Geometry: final body of the model. Coordinates: model frame, mm. A direction names the side the tool comes from. Coordinates: 2 decimals unless noted, no trailing zeros. Loops run counter-clockwise (first coordinate to the right, second up) from the corner with the lowest first, then second, coordinate; pieces in that order, holes last. Notation, with made-up numbers: (79, 87.25) - (130, 87.25) arc R20 cw to (130, 125.25) - close; hole circle Ø7 at (-20, 42.25). An arc over 180 degrees is marked (long way). Return JSON: item names as keys, results as strings.
Autodesk Inventor part; units mm, degrees
ref_plane "YZ Plane" through (0, 0, 0) normal (1, 0, 0) x (0, 1, 0)
ref_plane "XZ Plane" through (0, 0, 0) normal (0, 1, 0) x (-1, 0, 0)
ref_plane "XY Plane" through (0, 0, 0) normal (0, 0, 1) x (1, 0, 0)
sketch "Sketch1" plane through (0, 0, 0) normal (0, 0, 1) x (1, 0, 0)
  line L0 (-56, 0) -> (-28, 48.4974)
  line L1 (-28, 48.4974) -> (28, 48.4974)
  line L2 (28, 48.4974) -> (56, 0)
  line L3 (56, 0) -> (28, -48.4974)
  line L4 (28, -48.4974) -> (-28, -48.4974)
  line L5 (-28, -48.4974) -> (-56, 0)
  circle A0 centre (0, 30) radius 2.5
  circle A1 centre (-25.9808, 15) radius 2.5
  circle A2 centre (-25.9808, -15) radius 2.5
  circle A3 centre (0, -30) radius 2.5
  circle A4 centre (25.9808, -15) radius 2.5
  circle A5 centre (25.9808, 15) radius 2.5
  point P0 (0, 0)
  point P1 (0, 0)
  dimension "d0" = 112
  dimension "d1" = 5
  dimension "d2" = 30
  dimension "d5" = 360
extrude "Extrusion1" add sketch "Sketch1" along normal blind 5
sketch "Sketch2" plane through (0, 0, 5) normal (0, 0, 1) x (1, 0, 0)
  line L0 (28, 48.4974) -> (-28, 48.4974)
  line L1 (28, 48.4974) -> (128, 48.4974)
  line L2 (128, 48.4974) -> (128, -48.4974)
  line L3 (128, -48.4974) -> (28, -48.4974)
  circle A0 centre (25.9808, 15) radius 2.5
  circle A1 centre (25.9808, -15) radius 2.5
  line L4 (56, 0) -> (28, 48.4974)
  line L5 (28, -48.4974) -> (56, 0)
  line L6 (-28, -48.4974) -> (28, -48.4974)
  line L7 (28, -48.4974) -> (56, 0)
  line L8 (28, 48.4974) -> (56, 0)
  line L9 (28, -48.4974) -> (128, -48.4974)
  line L10 (28, 48.4974) -> (128, 48.4974)
  point P0 (0, 0)
  dimension "d10" = 100
extrude "Extrusion2" add sketch "Sketch2" against normal blind 5 contours L1 L2 L3 L5 L4
sketch "Sketch3" plane through (128, -48.4974, 5) normal (1, 0, 0) x (0, 0, -1)
  line L0 (0, 0) -> (0, 96.9948)
  line L1 (-58, 96.9948) -> (-30, 48.4974)
  line L2 (-30, 48.4974) -> (-58, 0)
  line L3 (-58, 0) -> (-114, 0)
  line L4 (-114, 0) -> (-142, 48.4974)
  line L5 (-142, 48.4974) -> (-114, 96.9948)
  line L6 (-114, 96.9948) -> (-58, 96.9948)
  line L7 (0, 0) -> (-58, 0)
  line L8 (-58, 0) -> (-58, 96.9948) construction
  line L9 (-58, 96.9948) -> (0, 96.9948)
  line L10 (0, 96.9948) -> (0, 0)
  circle A0 centre (-86, 78.4974) radius 2.5
  circle A1 centre (-111.9808, 63.4974) radius 2.5
  circle A2 centre (-111.9808, 33.4974) radius 2.5
  circle A3 centre (-86, 18.4974) radius 2.5
  circle A4 centre (-60.0192, 33.4974) radius 2.5
  circle A5 centre (-60.0192, 63.4974) radius 2.5
  line L11 (-58, 0) -> (-30, 48.4974)
  line L12 (-30, 48.4974) -> (-58, 96.9948)
  line L13 (-58, 96.9948) -> (0, 96.9948)
  line L14 (0, 48.4974) -> (0, 0)
  line L15 (-58, 0) -> (0, 0)
  circle A6 centre (-86, 48.4974) radius 22.5
  point P0 (5, 48.4974)
  dimension "d17" = 112
  dimension "d18" = 30
  dimension "d19" = 5
  dimension "d20" = 30
  dimension "d23" = 360
  dimension "d27" = 45
extrude "Extrusion3" add sketch "Sketch3" against normal blind 5
sketch "Sketch4" plane through (0, 0, 5) normal (0, 0, 1) x (1, 0, 0)
  circle A0 centre (0, 0) radius 22.5
  dimension "d28" = 45
extrude "Extrusion4" cut sketch "Sketch4" against normal through all
sketch "Sketch5" plane through (0, 0, 5) normal (0, 0, 1) x (1, 0, 0)
  circle A0 centre (0, 0) radius 22.5
  line L0 (123, -48.4974) -> (123, 48.4974) construction
  line L1 (123, 48.4974) -> (-28, 48.4974)
  line L2 (-28, 48.4974) -> (-56, 0)
  line L3 (-56, 0) -> (-28, -48.4974)
  line L4 (-28, -48.4974) -> (123, -48.4974)
  circle A1 centre (25.9808, 15) radius 2.5
  circle A2 centre (25.9808, -15) radius 2.5
  circle A3 centre (0, -30) radius 2.5
  circle A4 centre (-25.9808, -15) radius 2.5
  circle A5 centre (-25.9808, 15) radius 2.5
  circle A6 centre (0, 30) radius 2.5
  line L5 (-22.2265, 38.4974) -> (113, 38.4974)
  line L6 (113, 38.4974) -> (113, -38.4974) construction
  line L7 (113, -38.4974) -> (-22.2265, -38.4974)
  line L8 (-22.2265, -38.4974) -> (-44.453, 0)
  line L9 (-44.453, 0) -> (-22.2265, 38.4974)
  line L10 (113, 38.4974) -> (123, 38.4974)
  line L11 (123, -48.4974) -> (123, 48.4974)
  line L12 (123, 48.4974) -> (123, 38.4974)
  line L13 (113, -38.4974) -> (123, -38.4974)
  line L14 (123, -38.4974) -> (123, -48.4974)
  dimension "d31" = 10
extrude "Extrusion5" add sketch "Sketch5" along normal blind 15 contours L11 L10 L5 L9 L8 L7 L13 L4 L3 L2 L1
sketch "Sketch7" plane through (123, -48.4974, 5) normal (-1, 0, 0) x (0, 0, 1)
  circle A0 centre (86, 78.4974) radius 2.5
  circle A1 centre (111.9808, 63.4974) radius 2.5
  circle A2 centre (111.9808, 33.4974) radius 2.5
  circle A3 centre (86, 18.4974) radius 2.5
  circle A4 centre (60.0192, 33.4974) radius 2.5
  circle A5 centre (60.0192, 63.4974) radius 2.5
  circle A6 centre (86, 48.4974) radius 22.5
  line L0 (15, 96.9948) -> (15, 86.9948)
  line L1 (15, 86.9948) -> (0, 86.9948)
  line L2 (0, 10) -> (0, 86.9948)
  line L3 (0, 10) -> (15, 10)
  line L4 (15, 10) -> (15, 0)
  line L5 (15, 0) -> (114, 0)
  line L6 (114, 0) -> (142, 48.4974)
  line L7 (142, 48.4974) -> (114, 96.9948)
  line L8 (114, 96.9948) -> (15, 96.9948)
  line L9 (0, 55.9974) -> (15, 55.9974)
  line L10 (15, 55.9974) -> (15, 40.9974)
  line L11 (15, 40.9974) -> (0, 40.9974)
  line L12 (0, 40.9974) -> (0, 55.9974)
  point P0 (-5, 48.4974)
  point P1 (0, 48.4974)
  dimension "d34" = 15
extrude "Extrusion6" cut sketch "Sketch7" against normal through all contours L9 L10 L11 L2
sketch "Sketch8" plane through (128, -48.4974, 0) normal (1, 0, 0) x (0, 0, -1)
  line L0 (-5, 40.9974) -> (-20, 40.9974)
  line L1 (-20, 40.9974) -> (-20, 55.9974)
  line L2 (-20, 55.9974) -> (-5, 55.9974)
  line L3 (-5, 55.9974) -> (-5, 40.9974)
  circle A0 centre (-91, 78.4974) radius 2.5
  circle A1 centre (-116.9808, 63.4974) radius 2.5
  circle A2 centre (-116.9808, 33.4974) radius 2.5
  circle A3 centre (-91, 18.4974) radius 2.5
  circle A4 centre (-65.0192, 33.4974) radius 2.5
  circle A5 centre (-65.0192, 63.4974) radius 2.5
  circle A6 centre (-91, 48.4974) radius 22.5
  line L4 (-119, 0) -> (0, 0)
  line L5 (0, 96.9948) -> (0, 0)
  line L6 (0, 96.9948) -> (-119, 96.9948)
  line L7 (-119, 96.9948) -> (-147, 48.4974)
  line L8 (-147, 48.4974) -> (-119, 0)
  line L9 (-113.2265, 86.9948) -> (-10, 86.9948)
  line L10 (-10, 86.9948) -> (-10, 10) construction
  line L11 (-10, 10) -> (-113.2265, 10)
  line L12 (-113.2265, 10) -> (-135.453, 48.4974)
  line L13 (-135.453, 48.4974) -> (-113.2265, 86.9948)
  line L14 (-10, 86.9948) -> (0, 86.9948)
  line L15 (-10, 10) -> (0, 10)
  line L16 (0, 96.9948) -> (0, 0)
  point P0 (0, 48.4974)
  dimension "d37" = 10
extrude "Extrusion7" add sketch "Sketch8" along normal blind 15 contours L8 L7 L6 L5 L14 L9 L13 L12 L11 L15 L4
sketch "Sketch9" plane through (128, -38.4974, 0) normal (1, 0, 0) x (0, 0, -1)
  line L0 (0, 76.9948) -> (0, 86.9948)
  line L1 (0, 76.9948) -> (-5, 76.9948)
  line L2 (-5, 76.9948) -> (-5, -0.838)
  line L3 (-5, -0.838) -> (0, -0.838)
  line L4 (0, -0.838) -> (0, 76.9948)
  line L5 (-5, 45.9974) -> (-5, 30.9974)
  point P0 (0, 38.4974)
extrude "Extrusion8" add sketch "Sketch9" along normal blind 15
sketch "Sketch10" plane through (128, -7.5, 20) normal (1, 0, 0) x (0, 0, -1)
  circle A0 centre (7.5, 35) radius 2.5
  circle A1 centre (7.5, -20) radius 2.5
  line L0 (0, 15) -> (15, 15) construction
  line L1 (7.5, -20) -> (7.5, 35) construction
  line L2 (0, 0) -> (0, 15) construction
  point P0 (20, 7.5)
  point P1 (7.5, 15)
  point P2 (7.5, 7.5)
  point P3 (0, 7.5)
  dimension "d42" = 5
  dimension "d43" = 5
  dimension "d44" = 55
extrude "Extrusion9" cut sketch "Sketch10" against normal blind 20
sketch "Sketch12" plane through (-28, 48.4974, 20) normal (0, 1, 0) x (1, 0, 0)
  line L0 (151, 0) -> (151, -99) construction
  line L1 (151, -60) -> (91, 0)
  line L2 (151, 0) -> (5.7735, 0) construction
  line L3 (151, 15) -> (151, 0)
  line L4 (91, 0) -> (151, 0)
  line L5 (151, 0) -> (151, -60)
  point P0 (28, 20)
  dimension "d47" = 60
  dimension "d48" = 60
extrude "Extrusion10" add sketch "Sketch12" against normal blind 10
sketch "Sketch13" plane through (-28, -48.4974, 20) normal (0, -1, 0) x (1, 0, 0)
  line L0 (151, 60) -> (91, 0)
  line L1 (0, 0) -> (151, 0)
  line L2 (151, 0) -> (151, 99)
  line L3 (91, 0) -> (151, 0)
  line L4 (151, 60) -> (151, -15)
  line L5 (151, 60) -> (151, 0)
  point P0 (28, -20)
extrude "Extrusion11" add sketch "Sketch13" against normal blind 10
sketch "Sketch14" plane through (123, -48.4974, 5) normal (-1, 0, 0) x (0, 0, 1)
  circle A0 centre (86, 48.4974) radius 22.5
  line L0 (114, 96.9948) -> (142, 48.4974)
  line L1 (142, 48.4974) -> (114, 0)
  line L2 (114, 0) -> (58, 0)
  line L3 (58, 0) -> (30, 48.4974)
  line L4 (30, 48.4974) -> (58, 96.9948)
  line L5 (58, 96.9948) -> (114, 96.9948)
  line L6 (114, 96.9948) -> (142, 48.4974)
  point P0 (-5, 48.4974)
extrude "Extrusion12" cut sketch "Sketch14" along normal through all
sketch "Sketch16" plane through (143, -48.4974, 0) normal (1, 0, 0) x (0, 0, -1)
  circle A0 centre (-91, 48.4974) radius 22.5 construction
  circle A1 centre (-142, 48.4974) radius 2.5
  circle A2 centre (-116.5, 4.3301) radius 2.5
  circle A3 centre (-65.5, 4.3301) radius 2.5
  circle A4 centre (-40, 48.4974) radius 2.5
  circle A5 centre (-65.5, 92.6647) radius 2.5
  circle A6 centre (-116.5, 92.6647) radius 2.5
  point P0 (0, 48.4974)
  point P1 (-147, 48.4974)
  dimension "d55" = 5
  dimension "d56" = 5
  dimension "d59" = 360
extrude "Extrusion13" cut sketch "Sketch16" against normal through all
sketch "Sketch17" plane through (143, -48.4974, 0) normal (1, 0, 0) x (0, 0, -1)
  circle A0 centre (-142, 48.4974) radius 2.5
  circle A1 centre (-91, 48.4974) radius 22.5 construction
  circle A2 centre (-142, 48.4974) radius 6.5
  circle A3 centre (-116.5, 4.3301) radius 6.5
  circle A4 centre (-65.5, 4.3301) radius 6.5
  circle A5 centre (-40, 48.4974) radius 6.5
  circle A6 centre (-65.5, 92.6647) radius 6.5
  circle A7 centre (-116.5, 92.6647) radius 6.5
  point P0 (0, 48.4974)
  dimension "d63" = 13
  dimension "d66" = 360
extrude "Extrusion14" cut sketch "Sketch17" against normal blind 5 contours A0 | A2 | A3 | A4 | A5 | A6 | A7
sketch "Sketch18" plane through (0, 0, 20) normal (0, 0, 1) x (1, 0, 0)
  circle A0 centre (-51, 0) radius 2.5
  circle A1 centre (-25.5, -44.1673) radius 2.5
  circle A2 centre (25.5, -44.1673) radius 2.5
  circle A3 centre (51, 0) radius 2.5
  circle A4 centre (25.5, 44.1673) radius 2.5
  circle A5 centre (-25.5, 44.1673) radius 2.5
  point P0 (0, 0)
  point P1 (-56, 0)
  dimension "d70" = 5
  dimension "d71" = 5
  dimension "d74" = 360
extrude "Extrusion15" cut sketch "Sketch18" against normal through all
sketch "Sketch19" plane through (0, 0, 20) normal (0, 0, 1) x (1, 0, 0)
  circle A0 centre (-51, 0) radius 2.5
  circle A1 centre (-51, 0) radius 6.5
  circle A2 centre (-25.5, -44.1673) radius 6.5
  circle A3 centre (25.5, -44.1673) radius 6.5
  circle A4 centre (51, 0) radius 6.5
  circle A5 centre (25.5, 44.1673) radius 6.5
  circle A6 centre (-25.5, 44.1673) radius 6.5
  point P0 (0, 0)
  dimension "d78" = 13
  dimension "d81" = 360
extrude "Extrusion16" cut sketch "Sketch19" against normal blind 5 contours A0 | A1 | A2 | A3 | A4 | A5 | A6
sketch "Sketch20" plane through (0, 0, 5) normal (0, 0, 1) x (1, 0, 0)
  circle A0 centre (25.9808, -15) radius 2.5
  circle A1 centre (25.9808, 15) radius 2.5
  circle A2 centre (0, 30) radius 2.5
  circle A3 centre (-25.9808, 15) radius 2.5
  circle A4 centre (-25.9808, -15) radius 2.5
  circle A5 centre (0, -30) radius 2.5
  point P0 (0, 0)
extrude "Extrusion17" add sketch "Sketch20" against normal blind 5
sketch "Sketch21" plane through (123, -48.4974, 5) normal (-1, 0, 0) x (0, 0, 1)
  circle A0 centre (86, 78.4974) radius 2.5
  circle A1 centre (60.0192, 63.4974) radius 2.5
  circle A2 centre (60.0192, 33.4974) radius 2.5
  circle A3 centre (86, 18.4974) radius 2.5
  circle A4 centre (111.9808, 33.4974) radius 2.5
  circle A5 centre (111.9808, 63.4974) radius 2.5
  point P0 (-5, 48.4974)
extrude "Extrusion18" add sketch "Sketch21" against normal blind 5
equation "\"d29\" = d28"
properties part number "TARM03" material "ABS Plastic"
Item 1: Ray query, probe 1 along Y at (x, z) = (-25.5, 4.75); probe 2 along Y at (x, z) = (1, 12); probe 3 along Y at (x, z) = (132.5, 65.5). Return the intervals inside material, ascending. Write a range as from..to.
Worked out:
{"probe 1": "-48.5..-46.67, -41.67..41.67, 46.67..48.5", "probe 2": "-48.5..-38.5, 38.5..48.5", "probe 3": "-48.5..-46.67, -41.67..-38.5, 38.5..41.67, 46.67..48.5"}
Item 2: Section query D-D, the plane x = 79.5. Return loops of the section in (y, z), and give its area (3 significant figures).
Worked out:
{"outline": "(-48.5, 0) - (48.5, 0) - (48.5, 36.5) - (38.5, 36.5) - (38.5, 5) - (-38.5, 5) - (-38.5, 36.5) - (-48.5, 36.5) - close", "area": "1,110 mm^2"}
Item 3: First-contact query: pin 1 Ø8.5 at (x, y) = (-24, -43.5) entering from +Z; pin 2 Ø12.5 at (x, y) = (-48, -2) entering from +Z; pin 3 Ø12 at (x, y) = (25.5, -25.5) entering from +Z. Flat tips, straight axial feed; report the tip coordinate or a pass-through.
Worked out:
{"pin 1": "z = 15", "pin 2": "z = 20", "pin 3": "z = 5"}
Item 4: Section query B-B, the plane x = 51. Return loops of the section in (y, z).
Worked out:
{"outline": "(-48.5, 0) - (-2.5, 0) - (-2.5, 5) - (-38.5, 5) - (-38.5, 20) - (-48.5, 20) - close; (2.5, 0) - (48.5, 0) - (48.5, 20) - (38.5, 20) - (38.5, 5) - (2.5, 5) - close"}
Item 5: Mould query, pull axis X, two halves, no side actions, for faces 4 (the face through (143, 15, 128)), 5 (the face through (66, -38.497, 20)), 6 (the face through (-37, 15, 20)). Classes: +X half, -X half, draft (parallel to the pull), parting line (faces both ways), or undercut.
Worked out:
{"face 4": "+X half", "face 5": "undercut", "face 6": "draft"}
Item 6: Section query C-C, the plane z = 40. Return loops of the section in (x, y), and give its area (3 significant figures).
Worked out:
{"outline": "(83, -48.5) - (143, -48.5) - (143, -38.5) - (128, -38.5) - (128, -2.5) - (123, -2.5) - (123, -38.5) - (83, -38.5) - close; (83, 38.5) - (123, 38.5) - (123, 2.5) - (128, 2.5) - (128, 38.5) - (143, 38.5) - (143, 48.5) - (83, 48.5) - close", "area": "1,560 mm^2"}
Item 7: Section query A-A, the plane z = 12.5. Count the separate pieces of the cut face and the enclosed holes in it, and give its area (3 significant figures).
Worked out:
{"separate pieces": "3", "enclosed holes": "5", "area": "4,530 mm^2"}
Item 8: Reachability of faces 1 (the face through (-33.495, 18.979, 12.395)), 2 (the face through (130.605, 44.918, 114.115)), 3 (the face through (138, -41, 66)) from +Z, -Z, +X, -X, +Y, -Y: full face, straight path, thin tool, end or side. Return the list, or none.
Worked out:
{"face 1": "+Z", "face 2": "+X, -X", "face 3": "+X"}
